Can you work these out from the drawing? Everything is in mm from the part's minimum corner. A direction names the side the tool comes from. Round coordinates to 2 decimals unless told otherwise and drop trailing zeros. Loops run counter-clockwise (first coordinate to the right, second up) from the corner with the lowest first, then second, coordinate; pieces in that order, holes last. Notation, with made-up numbers: (24.25, 14.5) -> (46.25, 14.5) arc R10 ccw to (46.25, 30.5) -> close; hole circle Ø11 at (-10, 67.25). An arc over 180 degrees is marked (long way). Answer as a JSON object with one key per item and string values.
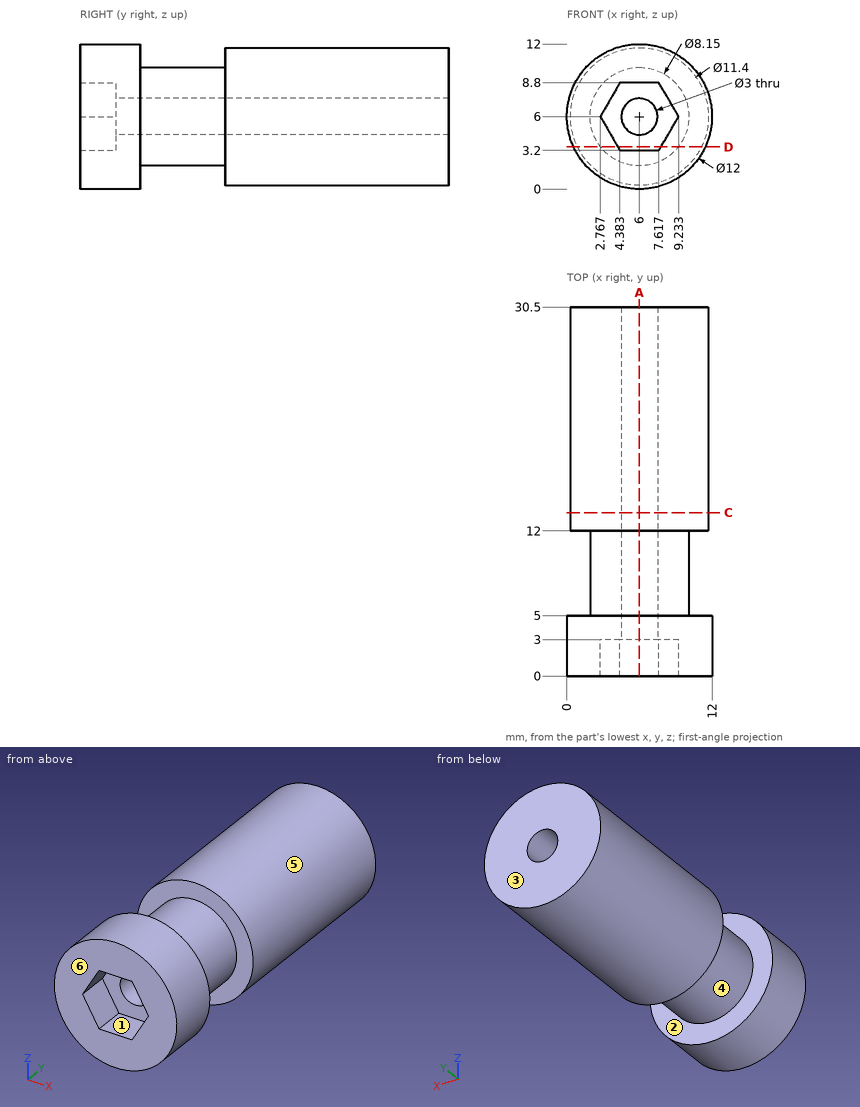
Q1. On a 3-axis mill with a long thin cutter (end or side, diameter ignored), from which of +Z, -Z, +X, -X, +Y, -Y can I reach the whole of each face in a straight line? I mean the marked faces 1, 2 and 3. Say none if no direction works.
Determined:
{"face 1": "-Y", "face 2": "none", "face 3": "+Z, -Z, +X, -X, +Y"}
Q2. I want a section at C-C, the plane y = 13.5. Write out the boundary of the cut face in (x, z).
Determined:
{"outline": "circle Ø11.4 at (6, 6); hole circle Ø3 at (6, 6)"}
Q3. We'd pull the mould along Y, two halves only. Please class the marked faces 4, 5 and 6: pulls with the +Y half, pulls with the -Y half, needs draft (parallel to the pull), parting line crosses it, or undercut.
Determined:
{"face 4": "undercut", "face 5": "needs draft", "face 6": "pulls with the -Y half"}
Q4. I want a section at D-D, the plane z = 3.5. Write out the boundary of the cut face in (x, y) (1 decimal).
Determined:
{"outline": "(0.5, 0) -> (4.2, 0) -> (4.2, 3) -> (7.8, 3) -> (7.8, 0) -> (11.5, 0) -> (11.5, 5) -> (9.2, 5) -> (9.2, 12) -> (11.1, 12) -> (11.1, 30.5) -> (0.9, 30.5) -> (0.9, 12) -> (2.8, 12) -> (2.8, 5) -> (0.5, 5) -> close"}
Q5. If I drill on L1, parallel to Y at x = 8.5, z = 1.75; L2, parallel to X at y = 20, z = 6; L3, parallel to Y at x = 6, z = 4.25, over which ranges is the centre line in solid material (lowest first)? Write a range as [from, to].
Determined:
{"L1": "[0, 5], [12, 30.5]", "L2": "[0.3, 4.5], [7.5, 11.7]", "L3": "[3, 30.5]"}
Q6. I'm going to push flat-ended pins straight in: pin 1 (1.5 mm diameter, centred on x = 3, y = 17, fed in from +Z); pin 2 (6 mm diameter, centred on y = 25.5, z = 9, fed in from +X); pin 3 (3 mm diameter, centred on y = 17.5, z = 8.5, fed in from -X). Where does each tip first touch, or does it pass through?
Determined:
{"pin 1": "z = 11.24", "pin 2": "x = 11.7", "pin 3": "x = 0.39"}
Q7. I want a section at A-A, the plane x = 6. Write out the boundary of the cut face in (y, z) (1 decimal).
Determined:
{"outline": "(0, 0) -> (5, 0) -> (5, 1.9) -> (12, 1.9) -> (12, 0.3) -> (30.5, 0.3) -> (30.5, 4.5) -> (3, 4.5) -> (3, 3.2) -> (0, 3.2) -> close; (0, 8.8) -> (3, 8.8) -> (3, 7.5) -> (30.5, 7.5) -> (30.5, 11.7) -> (12, 11.7) -> (12, 10.1) -> (5, 10.1) -> (5, 12) -> (0, 12) -> close"}
